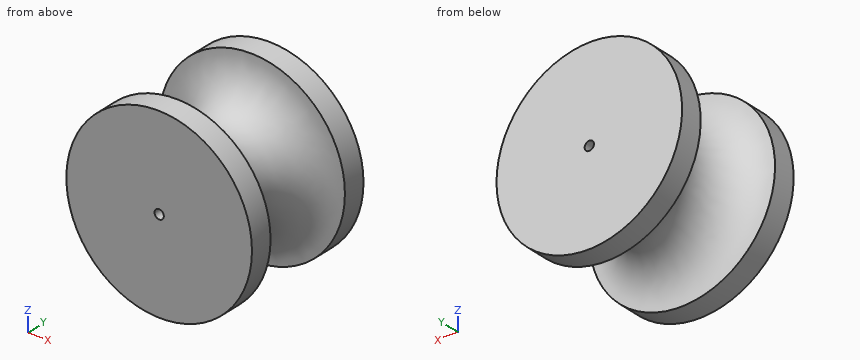
from build123d import *

# Parameters (mm, degrees)
F0_R     = 10
F1_DEPTH = 7.5
F5_R     = 0.5
F6_DEPTH = 15.001


with BuildPart() as f1:
    # F0 (on Front) → F1 (new body, symmetric)
    with BuildSketch(Plane.XZ):
        Circle(F0_R)
    extrude(amount=F1_DEPTH, both=True)

    # F2 (on Right) → F4 (revolve, cut)
    with BuildSketch(Plane.YZ):
        with BuildLine():
            Line((5, 10), (-5, 10))
            ThreePointArc((-5, 10), (0, 5), (5, 10))
        make_face()
    revolve(axis=Axis((0, -5.833439, 0), (0, 1, 0)), mode=Mode.SUBTRACT)

    # F5 (on face) → F6 (cut, through all)
    with BuildSketch(Plane.XZ.offset(7.5)):
        Circle(F5_R)
    extrude(amount=-F6_DEPTH, mode=Mode.SUBTRACT)


solid = f1.part
Can you work these out from the model? Positions are in its coordinate system, mm. Round coordinates to 2 decimals unless told otherwise and drop trailing zeros. Write each loop counter-clockwise with the first axis right and the second up, starting at its lowest first coordinate (ties: lowest second). Pieces come first, ordered by that corner, then holes. Notation, with made-up numbers: (36.5, 58.5) -> (49.5, 58.5) arc R28 ccw to (49.5, 77.5) -> close; hole circle Ø1 at (21, 37). An arc over 180 degrees is marked (long way). Use one line per item in the form item = value. Start each with the question number.
Q1. Imagine slicing it at A-A (x = 0). Please give me the cut outline in (y, z).
Q2. If I drill on probe 1 along Z at (x, y) = (0, 0); probe 2 along Y at (x, z) = (-1.5, 5.5); probe 3 along Y at (x, z) = (5.5, -2), over which ranges is the centre line in solid material (lowest first)? Write a range as [from, to].
Q3. Imagine slicing it at B-B (z = 0). Please give me the cut outline in (x, y), then the cut area to 3 significant figures.
Q4. I'm going to push flat-ended pins straight in: P1, Ø3, axis at x = 3, y = -5.5, coming from the -Z side; P2, Ø1, axis at x = -3.5, y = 0, coming from the -Z side; P3, Ø3, axis at y = 4.5, z = 5.5, coming from the +X side. Where does each tip first touch, or does it pass through?
Q5. Imagine slicing it at C-C (y = -6.25). Please give me the cut outline in (x, z).
Q6. Imagine slicing it at D-D (y = 1.75). Please give me the cut outline in (x, z), then the cut area to 3 significant figures.
Worked out:
q1.outline = (-7.5, -10) -> (-5, -10) arc R5 cw to (5, -10) -> (7.5, -10) -> (7.5, -0.5) -> (-7.5, -0.5) -> close; (-7.5, 0.5) -> (7.5, 0.5) -> (7.5, 10) -> (5, 10) arc R5 cw to (-5, 10) -> (-7.5, 10) -> close
q2.probe_1 = [-5, -0.5], [0.5, 5]
q2.probe_2 = [-7.5, -2.55], [2.55, 7.5]
q2.probe_3 = [-7.5, -2.79], [2.79, 7.5]
q3.outline = (-10, -7.5) -> (-0.5, -7.5) -> (-0.5, 7.5) -> (-10, 7.5) -> (-10, 5) arc R5 cw to (-10, -5) -> close; (0.5, -7.5) -> (10, -7.5) -> (10, -5) arc R5 cw to (10, 5) -> (10, 7.5) -> (0.5, 7.5) -> close
q3.area = 206 mm^2
q4.P1 = -9.89
q4.P2 = -4
q4.P3 = 9.13
q5.outline = circle Ø20 at (0, 0); hole circle Ø1 at (0, 0)
q6.outline = circle Ø10.63 at (0, 0); hole circle Ø1 at (0, 0)
q6.area = 88.0 mm^2
